```python
from build123d import *

# Parameters (mm, degrees)
BOSS_EXTRUDE2_DEPTH       = 1.6
SKETCH3_R                 = 1.7
CUT_EXTRUDE1_DEPTH        = 2.6
CIRPATTERN1_COUNT         = 3
SKETCH4_W                 = 13.934293336
SKETCH4_H                 = 5.4356
BOSS_EXTRUDE3_DEPTH       = 11.5
SKETCH5_W                 = 6.096
SKETCH5_H                 = 8.5
BOSS_EXTRUDE4_DEPTH       = 13.1191
CHAMFER1_SIZE             = 2
CHAMFER1_SIZE2            = 3.464101615
CHAMFER1_OF_MIRROR1_SIZE2 = 2
CHAMFER1_OF_MIRROR1_SIZE  = 3.464101615
SKETCH6_W                 = 22
SKETCH6_H                 = 4.4356
CUT_EXTRUDE2_DEPTH        = 13.434293
SKETCH8_W                 = 6.096
SKETCH8_H                 = 13.1191
BOSS_EXTRUDE5_DEPTH       = 2


with BuildPart() as part:
    # Sketch2 → Boss-Extrude2 (new body)
    with BuildSketch(Plane(origin=(0, 0, 0), x_dir=(1, 0, 0), z_dir=(0, 1, 0))):
        with BuildLine():
            ThreePointArc((5.974383185, -31.946153846), (0, 32.5), (-5.974383185, -31.946153846))
            ThreePointArc((-5.974383185, -31.946153846), (0, -26.5), (5.974383185, -31.946153846))
        make_face()
    extrude(amount=BOSS_EXTRUDE2_DEPTH)

    # Sketch3 → Cut-Extrude1 (cut, through all)
    with BuildSketch(Plane(origin=(0, 1.6, 0), x_dir=(1, 0, 0), z_dir=(0, 1, 0))):
        with Locations((10.301681319, -25.497556001)):
            Circle(SKETCH3_R)
    cut_extrude1 = extrude(amount=-CUT_EXTRUDE1_DEPTH, mode=Mode.SUBTRACT)

    # CirPattern1: Cut-Extrude1 ×3 about axis
    cirpattern1_axis = Axis((0, 0, 0), (0, 1, 0))
    for i in range(1, CIRPATTERN1_COUNT):
        add(cut_extrude1.rotate(cirpattern1_axis, i * 360 / CIRPATTERN1_COUNT), mode=Mode.SUBTRACT)

    # Sketch4 → Boss-Extrude3 (add, symmetric)
    with BuildSketch(Plane(origin=(0, 0, 0), x_dir=(0, 0, -1), z_dir=(1, 0, 0))):
        with Locations((19.967146668, 4.3178)):
            Rectangle(SKETCH4_W, SKETCH4_H)
    extrude(amount=BOSS_EXTRUDE3_DEPTH, both=True)

    # Sketch5 → Boss-Extrude4 (add)
    with BuildSketch(Plane.XY.offset(7.6)):
        with Locations((15.848, 5.85)):
            Rectangle(SKETCH5_W, SKETCH5_H)
    boss_extrude4 = extrude(amount=BOSS_EXTRUDE4_DEPTH)

    # Chamfer1
    chamfer1_edges = [part.edges().sort_by_distance(p)[0] for p in [
        (12.8, 10.1, 14.15955),
        (18.896, 10.1, 14.15955),
    ]]
    chamfer1_side = [part.faces().sort_by_distance(p)[0] for p in [
        (15.848, 10.1, 14.15955),
    ]]
    chamfer(chamfer1_edges, length=CHAMFER1_SIZE, length2=CHAMFER1_SIZE2, reference=chamfer1_side[0])

    # Mirror1: Boss-Extrude4 across plane
    add(boss_extrude4.mirror(Plane(origin=(0, 0, 0), x_dir=(0, 0, 1), z_dir=(1, 0, 0))))

    # Chamfer1 of Mirror1
    chamfer1_of_mirror1_edges = [part.edges().sort_by_distance(p)[0] for p in [
        (-12.8, 10.1, 14.15955),
        (-18.896, 10.1, 14.15955),
    ]]
    chamfer(chamfer1_of_mirror1_edges, length=CHAMFER1_OF_MIRROR1_SIZE, length2=CHAMFER1_OF_MIRROR1_SIZE2)

    # Sketch6 → Cut-Extrude2 (cut)
    with BuildSketch(Plane.XY.offset(-13)):
        with Locations((0, 4.3178)):
            Rectangle(SKETCH6_W, SKETCH6_H)
    extrude(amount=-CUT_EXTRUDE2_DEPTH, mode=Mode.SUBTRACT)

    # Sketch8 → Boss-Extrude5 (add)
    with BuildSketch(Plane.XZ):
        with Locations((15.848, 14.15955)):
            Rectangle(SKETCH8_W, SKETCH8_H)
        with Locations((-15.848, 14.15955)):
            Rectangle(SKETCH8_W, SKETCH8_H)
    extrude(amount=BOSS_EXTRUDE5_DEPTH)


solid = part.part
```
CAD build for the part. Positions are in the model's coordinates, mm. A direction names the side the tool comes from. Give positions to 0.01 mm unless a question says otherwise; leave off trailing zeros. Order: outer loops, then holes, each group sorted by start corner. A loop starts at its lowest first (then second) coordinate and runs counter-clockwise, first axis right, second up. Notation, with made-up numbers: M 68.5,-25 L 109.5,-25 A25 ccw 109.5,-1 Z; hole C 26,60 d5. An arc over 180 degrees is marked long. Put each result on its own line as item: value. Start each with the question number.
(1) Saw through at A-A, the plane y = 5. Write the cut outline in (x, z).
(2) Saw through at D-D, the plane z = -22. Write the cut outline in (x, y), then the cut area to 3 significant figures.
(3) Mould opens along Y. For faces 4 (the flat face through (11, 4, -20)), 5 (the flat face through (-11, 4, -20)), 6 (the flat face through (-12.8, 4, 14)), 7 (the flat face through (-16, 10.1, 14)) say: +Y half, -Y half, draft (parallel to the pull), parting line (faces both ways), or undercut.
(4) Which spindle directions (+Z, -Z, +X, -X, +Y, -Y) get a long thin tool onto all of the face, cutting with end or side? Do faces 1 (the flat face through (0, 4, -26.434)), 2 (the flat face through (0, 4, -26.934)), 3 (the flat face through (12.8, -1, 14)). Say none if no direction does.
(5) Flat gauge pins, fed straight in: pin 1 Ø4 at (y, z) = (4.5, 15.5) entering from +X; pin 2 Ø4 at (x, z) = (-0.5, -17) entering from +Y; pin 3 Ø4 at (x, y) = (1.5, 9) entering from +Z. Where does each tip first touch, or does it go through?
(6) Saw through at B-B, the plane z = 28. Write the cut outline in (x, y), then the cut area to 3 significant figures.
(7) Saw through at C-C, the plane y = -0.75. Write the cut outline in (x, z).
(8) Drill centre lines: line 1 along X through (y, z) = (6.5, 9); line 2 along X through (y, z) = (6, -21); line 3 along Y through (x, z) = (-5, -26). Where is each one in solid material? Low to high.
Check result:
1. outline: M -18.9,7.6 L -12.8,7.6 L -12.8,20.72 L -18.9,20.72 Z; M -11.5,-26.93 L 11.5,-26.93 L 11.5,-13 L 11,-13 L 11,-26.43 L -11,-26.43 L -11,-13 L -11.5,-13 Z; M 12.8,7.6 L 18.9,7.6 L 18.9,20.72 L 12.8,20.72 Z
2. outline: M -23.92,0 L 15.26,0 L 15.26,1.6 L 11.5,1.6 L 11.5,7.04 L -11.5,7.04 L -11.5,1.6 L -23.92,1.6 Z; M 18.6,0 L 23.92,0 L 23.92,1.6 L 18.6,1.6 Z; hole M -11,2.1 L 11,2.1 L 11,6.54 L -11,6.54 Z
2. area: 98.6 mm2
3. face 4: undercut
3. face 5: undercut
3. face 6: draft
3. face 7: +Y half
4. face 1: +Z
4. face 2: -Z, +X, -X, +Y
4. face 3: +Z, -Z, -Y
5. pin 1: stops at x = 18.9
5. pin 2: stops at y = 7.04
5. pin 3: stops at z = -13
6. outline: M -16.5,0 L -3.97,0 L -3.97,1.6 L -16.5,1.6 Z; M 3.97,0 L 16.5,0 L 16.5,1.6 L 3.97,1.6 Z
6. area: 40.1 mm2
7. outline: M -18.9,7.6 L -12.8,7.6 L -12.8,20.72 L -18.9,20.72 Z; M 12.8,7.6 L 18.9,7.6 L 18.9,20.72 L 12.8,20.72 Z
8. line 1: x = -18.9 to -12.8, 12.8 to 18.9
8. line 2: x = -11.5 to -11, 11 to 11.5
8. line 3: y = 0 to 2.1, 6.54 to 7.04
